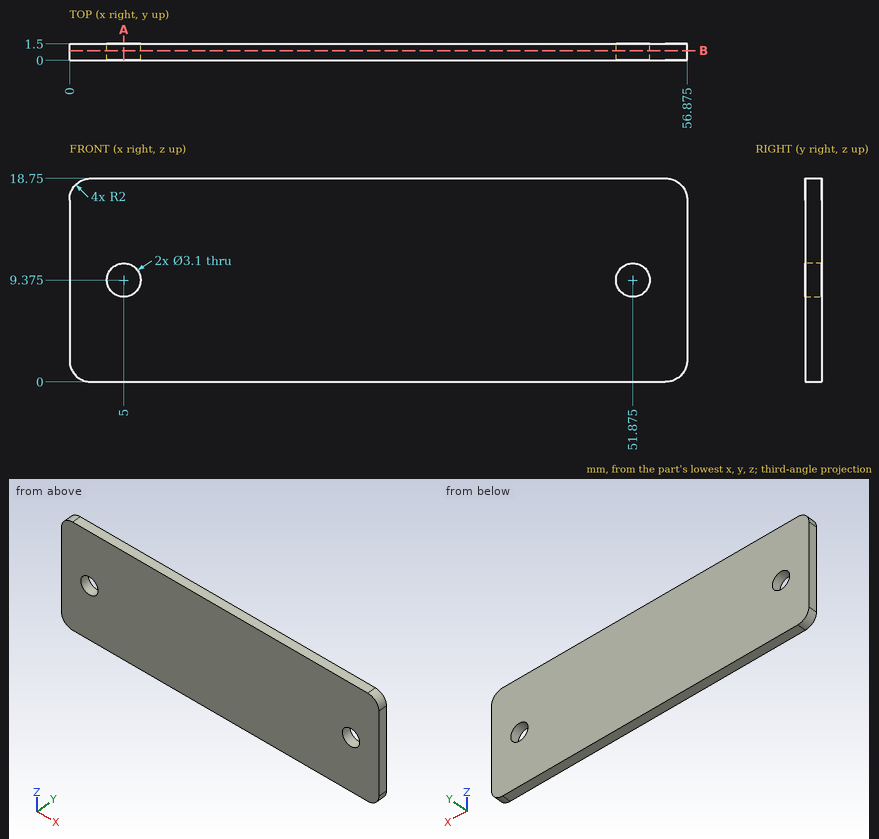
Answer from the drawing. Dimensions are ordinates in mm from the lowest x, y and z of the part. Round coordinates to 2 decimals unless told otherwise and drop trailing zeros. Order: outer loops, then holes, each group sorted by start corner. A loop starts at its lowest first (then second) coordinate and runs counter-clockwise, first axis right, second up. Notation, with made-up numbers: (51, -26.5) - (82, -26.5) arc R27 cw to (82, 5.5) - close; hole circle Ø11 at (60, -23.75). An arc over 180 degrees is marked (long way). Put each result on its own line as item: value. Start each with the question number.
(1) Find section B-B (y = 0.9). Give the vertices of the cut face in (x, z) (3 decimals).
(2) Straight lines are drawn through the part: probe 1 along X at (y, z) = (0.45, 10.5) (3 decimals); probe 2 along X at (y, z) = (1.1, 10.25) (3 decimals); probe 3 along X at (y, z) = (1.25, 1.25). For each, find the intervals that lie inside material, in ascending order. Write a range as from..to.
(3) Given P1, Ø3, axis at x = 51.875, z = 9.375, coming from the +Y side, flat-ended and moving along its own axis, determine where the tip first touches the part or whether it passes through.
(4) Find section A-A (x = 5). Give the vertices of the cut face in (y, z) (3 decimals), plus the area to 3 significant figures.
Reply:
1. outline: (0, 2) arc R2 ccw to (2, 0) - (54.875, 0) arc R2 ccw to (56.875, 2) - (56.875, 16.75) arc R2 ccw to (54.875, 18.75) - (2, 18.75) arc R2 ccw to (0, 16.75) - close; hole circle Ø3.1 at (5, 9.375); hole circle Ø3.1 at (51.875, 9.375)
2. probe 1: 0..3.934, 6.066..50.809, 52.941..56.875
2. probe 2: 0..3.721, 6.279..50.596, 53.154..56.875
2. probe 3: 0.15..56.73
3. P1: through
4. outline: (0, 0) - (1.5, 0) - (1.5, 7.825) - (0, 7.825) - close; (0, 10.925) - (1.5, 10.925) - (1.5, 18.75) - (0, 18.75) - close
4. area: 23.5 mm^2
